```python
from build123d import *

# Parameters (mm, degrees)
F1_DEPTH = 15
F2_SIZE  = 10


with BuildPart() as f1:
    # F0 (on Front) → F1 (new body)
    with BuildSketch(Plane.XZ):
        Polygon((17.871871, 80), (-25, -80), (25, -80), (25, 80), align=None)
    extrude(amount=F1_DEPTH)

    # F2
    f2_edges = [f1.edges().sort_by_distance(p)[0] for p in [
        (25, -7.5, -80),
    ]]
    chamfer(f2_edges, length=F2_SIZE)


solid = f1.part
```
Geometry: final body of the model. Coordinates: model frame, mm. Give positions to 0.01 mm unless a question says otherwise; leave off trailing zeros. Order: outer loops, then holes, each group sorted by start corner. A loop starts at its lowest first (then second) coordinate and runs counter-clockwise, first axis right, second up. Notation, with made-up numbers: M 68,20 L 79,20 A34 cw 79,58 Z; hole C -18.5,33 d1. An arc over 180 degrees is marked long. Answer as CSV lines item,"result". Start each with the question number.
1) Line query: line 1 (X direction, y = -1, z = 6); line 2 (X direction, y = -11, z = 12.5). Output: solid intervals per line, ascending. Write a range as from..to.
2) First-contact query: P1, Ø4, axis at y = -10.5, z = 51, coming from the -X side. Flat tip, straight axial feed; report the tip coordinate or a pass-through.
3) Cut plane A-A (y = -12.25). Output: boundary loops of the cut face in (x, z).
4) Cut plane B-B (z = -54). Output: boundary loops of the cut face in (x, y), then the cut area to 4 significant figures.
5) Cut plane C-C (x = 7). Output: boundary loops of the cut face in (y, z).
Findings below:
1,line 1,"x = -1.96..25"
1,line 2,"x = -0.21..25"
2,P1,"stops at x = 9.57"
3,outline,"M -25,-80 L 15,-80 L 25,-70 L 25,80 L 17.87,80 Z"
4,outline,"M -18.03,-15 L 25,-15 L 25,0 L -18.03,0 Z"
4,area,"645.5 mm²"
5,outline,"M -15,-80 L 0,-80 L 0,39.43 L -15,39.43 Z"
